Build history of the part. All positions in model axes, mm. A direction names the side the tool comes from. Round coordinates to 2 decimals unless told otherwise and drop trailing zeros. Order: outer loops, then holes, each group sorted by start corner. A loop starts at its lowest first (then second) coordinate and runs counter-clockwise, first axis right, second up. Notation, with made-up numbers: (-25.75, 71) -> (13.25, 71) arc R8 ccw to (13.25, 84) -> close; hole circle Ø3 at (10.25, 51.25). An arc over 180 degrees is marked (long way). Use a Markdown table: item, result. Add a question column.
Item 1: Slice it at B-B, the plane y = -10. Give the cut face in (x, z), plus the area to 3 significant figures.
Item 2: Slice it at C-C, the plane x = -16.5. Give the cut face in (y, z).
Item 3: Two-plate mould, pull along Z, no slides. Class faces 6 (the face through (20, 5, 0)), 7 (the face through (0, -18.8, 0)), 8 (the face through (-16, 5, 10)): released by +Z, released by -Z, zero draft, split by the parting line, or undercut.
Item 4: Probe L1, parallel to X at y = -13.75, z = 0; L2, parallel to Y at x = -16, z = 4.5; L3, parallel to X at y = 6.5, z = -3.5. List the from-to ranges inside material, lowest first.
Item 5: Pin check, flat tips, straight feed: pin 1 (7 mm diameter, centred on x = -13.5, y = 3.5, fed in from +Z); pin 2 (7 mm diameter, centred on x = 15, y = 4, fed in from +Z); pin 3 (9.5 mm diameter, centred on x = 16, y = 6.5, fed in from -Z). Stop position of each tip, or through.
Item 6: Slice it at A-A, the plane z = 0. Give the cut face in (x, y).
Item 7: Slice it at D-D, the plane y = -24. Give the cut face in (x, z).
Item 8: 3-axis set-ups, long thin cutter, end or side, ignore diameter. For faces 1 (the face through (16, 5, 10)), 2 (the face through (16, 5, -10)), 3 (the face through (-16, 5, -10)), 4 (the face through (7.27, -13.85, 7.92)), 5 (the face through (0.165, -6.226, -3.746)): which of +Z, -Z, +X, -X, +Y, -Y reach the whole face in a straight line?
from build123d import *

# Parameters (mm, degrees)
SKETCH1_R           = 15
BOSS_EXTRUDE1_DEPTH = 10
SKETCH2_R           = 10.75
BOSS_EXTRUDE2_DEPTH = 25
SKETCH3_R           = 3.75
CUT_EXTRUDE1_DEPTH  = 28.8
SKETCH5_R           = 10.75
BOSS_EXTRUDE4_DEPTH = 10
BOSS_EXTRUDE4_TAPER = 25
CHAMFER1_SIZE       = 4
BOSS_EXTRUDE3_START = -10
SKETCH4_R           = 7.75
BOSS_EXTRUDE3_DEPTH = 10
FILLET1_R           = 3


with BuildPart() as part:
    # Sketch1 → Boss-Extrude1 (new body)
    with BuildSketch(Plane(origin=(0, 0, 0), x_dir=(1, 0, 0), z_dir=(0, 1, 0))):
        with Locations(Location((0, 0, 0), (0, 0, 270))):
            Circle(SKETCH1_R)
    extrude(amount=BOSS_EXTRUDE1_DEPTH)

    # Sketch2 → Boss-Extrude2 (add)
    with BuildSketch(Plane.XZ):
        with Locations(Location((0, 0, 0), (0, 0, 270))):
            Circle(SKETCH2_R)
    extrude(amount=BOSS_EXTRUDE2_DEPTH)

    # Sketch3 → Cut-Extrude1 (cut)
    with BuildSketch(Plane(origin=(0, 10, 0), x_dir=(1, 0, 0), z_dir=(0, 1, 0))):
        with Locations(Location((0, 0, 0), (0, 0, 270))):
            Circle(SKETCH3_R)
    extrude(amount=-CUT_EXTRUDE1_DEPTH, mode=Mode.SUBTRACT)

    # Sketch5 → Boss-Extrude4 (add)
    with BuildSketch(Plane.XZ.offset(25)):
        with Locations(Location((0, 0, 0), (0, 0, 270))):
            Circle(SKETCH5_R)
    extrude(amount=BOSS_EXTRUDE4_DEPTH, taper=BOSS_EXTRUDE4_TAPER)

    # Chamfer1
    chamfer1_edges = [part.edges().sort_by_distance(p)[0] for p in [
        (0, 10, -3.75),
    ]]
    chamfer(chamfer1_edges, length=CHAMFER1_SIZE)

    # Sketch4 → Boss-Extrude3 (add)
    # profile 1 of 3: a face of its own
    with BuildSketch(Plane(origin=(0, 10, 0), x_dir=(1, 0, 0), z_dir=(0, 1, 0)).offset(BOSS_EXTRUDE3_START)):
        with BuildLine():
            Line((-11.180339887, 10), (-20, 10))
            Line((-20, 10), (-20, -10))
            Line((-20, -10), (-11.180339887, -10))
            ThreePointArc((-11.180339887, -10), (-15, 0), (-11.180339887, 10))
        make_face()
    # profile 2 of 3: a face of its own
    with BuildSketch(Plane(origin=(0, 10, 0), x_dir=(1, 0, 0), z_dir=(0, 1, 0)).offset(BOSS_EXTRUDE3_START)):
        with BuildLine():
            Line((11.180339887, 10), (-11.180339887, 10))
            ThreePointArc((-11.180339887, 10), (-15, 0), (-11.180339887, -10))
            Line((-11.180339887, -10), (11.180339887, -10))
            ThreePointArc((11.180339887, -10), (14.012585384, -5.352331347), (15, 0))
            ThreePointArc((15, 0), (14.012585384, 5.352331347), (11.180339887, 10))
        make_face()
        Circle(SKETCH4_R, mode=Mode.SUBTRACT)
    # profile 3 of 3: a face of its own
    with BuildSketch(Plane(origin=(0, 10, 0), x_dir=(1, 0, 0), z_dir=(0, 1, 0)).offset(BOSS_EXTRUDE3_START)):
        with BuildLine():
            Line((20, 10), (11.180339887, 10))
            ThreePointArc((11.180339887, 10), (14.012585384, 5.352331347), (15, 0))
            ThreePointArc((15, 0), (14.012585384, -5.352331347), (11.180339887, -10))
            Line((11.180339887, -10), (20, -10))
            Line((20, -10), (20, 10))
        make_face()
    extrude(amount=BOSS_EXTRUDE3_DEPTH)

    # Fillet1
    fillet1_edges = [part.edges().sort_by_distance(p)[0] for p in [
        (0, 0, 10.75),
    ]]
    fillet(fillet1_edges, radius=FILLET1_R)


solid = part.part
Check sheet entries:
| question | item | result |
|---|---|---|
| 1 | outline | circle Ø21.5 at (0, 0); hole circle Ø7.5 at (0, 0) |
| 1 | area | 319 mm2 |
| 2 | outline | (0, -10) -> (10, -10) -> (10, 10) -> (0, 10) -> close |
| 3 | face 6 | zero draft |
| 3 | face 7 | undercut |
| 3 | face 8 | released by +Z |
| 4 | L1 | -10.75 to -3.75, 3.75 to 10.75 |
| 4 | L2 | 0 to 10 |
| 4 | L3 | -20 to -2.41, 2.41 to 20 |
| 5 | pin 1 | z = 11.18 |
| 5 | pin 2 | z = 10 |
| 5 | pin 3 | z = -10 |
| 6 | outline | (-20, 0) -> (-13.75, 0) arc R3 cw to (-10.75, -3) -> (-10.75, -25) -> (-6.09, -35) -> (6.09, -35) -> (10.75, -25) -> (10.75, -3) arc R3 cw to (13.75, 0) -> (20, 0) -> (20, 10) -> (7.75, 10) -> (3.75, 6) -> (3.75, -18.8) -> (-3.75, -18.8) -> (-3.75, 6) -> (-7.75, 10) -> (-20, 10) -> close |
| 7 | outline | circle Ø21.5 at (0, 0) |
| 8 | face 1 | +Z, +X, +Y, -Y |
| 8 | face 2 | -Z, +X, +Y, -Y |
| 8 | face 3 | -Z, -X, +Y, -Y |
| 8 | face 4 | -Y |
| 8 | face 5 | +Y |
